The model under review builds one solid part; all positions refer to its coordinate system, in mm. Face numbers are marked on the shaded views. A direction names the side the tool comes from. Round coordinates to 2 decimals unless told otherwise and drop trailing zeros. Order: outer loops, then holes, each group sorted by start corner. A loop starts at its lowest first (then second) coordinate and runs counter-clockwise, first axis right, second up. Notation, with made-up numbers: (-39.5, 7) -> (17.5, 7) arc R12 ccw to (17.5, 20) -> close; hole circle Ø8 at (-34, 4.5). An arc over 180 degrees is marked (long way). Return JSON: item names as keys, results as strings. Group by question number.
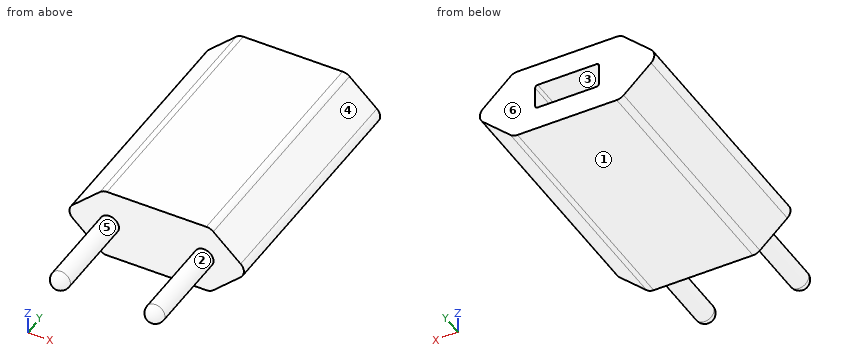
from build123d import *

# Parameters (mm, degrees)
F1_DEPTH = 24
F2_R     = 1.875
F3_DEPTH = 19
F4_R     = 1.875
F6_DEPTH = 11.5


with BuildPart() as f1:
    # F0 (on Front) → F1 (new body, symmetric)
    with BuildSketch(Plane.XZ):
        with BuildLine():
            Line((-11.07631, 6.462111), (-16.433453, 1.462111))
            ThreePointArc((-16.433453, 1.462111), (-17.068816, 0), (-16.433453, -1.462111))
            Line((-16.433453, -1.462111), (-11.07631, -6.462111))
            ThreePointArc((-11.07631, -6.462111), (-10.445083, -6.860675), (-9.711674, -7))
            Line((-9.711674, -7), (9.711674, -7))
            ThreePointArc((9.711674, -7), (10.445083, -6.860675), (11.07631, -6.462111))
            Line((11.07631, -6.462111), (16.433453, -1.462111))
            ThreePointArc((16.433453, -1.462111), (17.068816, 0), (16.433453, 1.462111))
            Line((16.433453, 1.462111), (11.07631, 6.462111))
            ThreePointArc((11.07631, 6.462111), (10.445083, 6.860675), (9.711674, 7))
            Line((9.711674, 7), (-9.711674, 7))
            ThreePointArc((-9.711674, 7), (-10.445083, 6.860675), (-11.07631, 6.462111))
        make_face()
    extrude(amount=F1_DEPTH, both=True)

    # F2 (on face) → F3 (join)
    with BuildSketch(Plane.XZ.offset(24)):
        with Locations((-9.25, 0)):
            Circle(F2_R)
        with Locations((9.25, 0)):
            Circle(F2_R)
    extrude(amount=F3_DEPTH)

    # F4
    f4_edges = [f1.edges().sort_by_distance(p)[0] for p in [
        (-11.125, -43, 0),
        (7.375, -43, 0),
    ]]
    fillet(f4_edges, radius=F4_R)

    # F5 (on face) → F6 (cut)
    with BuildSketch(Plane(origin=(0, 24, 0), x_dir=(-1, 0, 0), z_dir=(0, 1, 0))):
        with BuildLine():
            ThreePointArc((6.25, 2), (6.103553, 2.353553), (5.75, 2.5))
            Line((5.75, 2.5), (-5.75, 2.5))
            ThreePointArc((-5.75, 2.5), (-6.103553, 2.353553), (-6.25, 2))
            Line((-6.25, 2), (-6.25, -2))
            ThreePointArc((-6.25, -2), (-6.103553, -2.353553), (-5.75, -2.5))
            Line((-5.75, -2.5), (5.75, -2.5))
            ThreePointArc((5.75, -2.5), (6.103553, -2.353553), (6.25, -2))
            Line((6.25, -2), (6.25, 2))
        make_face()
    extrude(amount=-F6_DEPTH, mode=Mode.SUBTRACT)


solid = f1.part
Item 1: Insertion check: pin 1 Ø1 at (x, z) = (9.5, 3) entering from -Y; pin 2 Ø2 at (x, y) = (10, -28.5) entering from -Z (3 decimals); pin 3 Ø2.5 at (x, z) = (2.5, 0) entering from +Y. Each pin has a flat end and moves straight along its axis. Give the tip position at first contact, or say it passes through.
Item 2: The part is to be moulded in two halves that separate along X. For the marked faces 4, 5 and 6, say which applies: +X half, -X half, draft (parallel to the pull), parting line (faces both ways), or undercut.
Item 3: Consider section B-B on x = 3.5. State the section outline as (y, z) points, plus the area to 4 significant figures.
Item 4: Wall thickness on line 1 along Y through (x, z) = (15, 1.25); line 2 along X through (y, z) = (-31, -1.5) (3 decimals); line 3 along X through (y, z) = (15.5, 0.75): over which ranges is each line inside the solid? List them lowest first.
Item 5: Consider section D-D on x = -8. State the section outline as (y, z) points (3 decimals).
Item 6: Consider section C-C on y = -14.5. State the section outline as (x, z) points, plus the area to 3 significant figures.
Item 7: For the marked faces 1, 2 and 3, list the 3-axis set-ups (+Z, -Z, +X, -X, +Y, -Y) from which the entire face can be reached by the end or side of a thin tool; tool diameter is ignored.
Item 8: Consider section A-A on z = 0. State the section outline as (x, y) points (3 decimals), plus the area to 3 significant figures.
Values:
{
 "1": {"pin 1": "y = -24", "pin 2": "z = -1.875", "pin 3": "y = 12.5"},
 "2": {"face 4": "+X half", "face 5": "undercut", "face 6": "draft"},
 "3": {"outline": "(-24, -7) -> (24, -7) -> (24, -2.5) -> (12.5, -2.5) -> (12.5, 2.5) -> (24, 2.5) -> (24, 7) -> (-24, 7) -> close", "area": "614.5 mm^2"},
 "4": {"line 1": "-24 to 24", "line 2": "-10.375 to -8.125, 8.125 to 10.375", "line 3": "-16.92 to -6.25, 6.25 to 16.92"},
 "5": {"outline": "(-41.125, -1.398) -> (-24, -1.398) -> (-24, -7) -> (24, -7) -> (24, 7) -> (-24, 7) -> (-24, 1.398) -> (-41.125, 1.398) arc R1.398 ccw to start"},
 "6": {"outline": "(-16.43, -1.46) -> (-11.08, -6.46) arc R2 ccw to (-9.71, -7) -> (9.71, -7) arc R2 ccw to (11.08, -6.46) -> (16.43, -1.46) arc R2 ccw to (16.43, 1.46) -> (11.08, 6.46) arc R2 ccw to (9.71, 7) -> (-9.71, 7) arc R2 ccw to (-11.08, 6.46) -> (-16.43, 1.46) arc R2 ccw to start", "area": "397 mm^2"},
 "7": {"face 1": "-Z, +X, -X, +Y, -Y", "face 2": "-Y", "face 3": "+Y"},
 "8": {"outline": "(-17.069, -24) -> (-11.125, -24) -> (-11.125, -41.125) arc R1.875 ccw to (-7.375, -41.125) -> (-7.375, -24) -> (7.375, -24) -> (7.375, -41.125) arc R1.875 ccw to (11.125, -41.125) -> (11.125, -24) -> (17.069, -24) -> (17.069, 24) -> (6.25, 24) -> (6.25, 12.5) -> (-6.25, 12.5) -> (-6.25, 24) -> (-17.069, 24) -> close", "area": "1,630 mm^2"}
}
